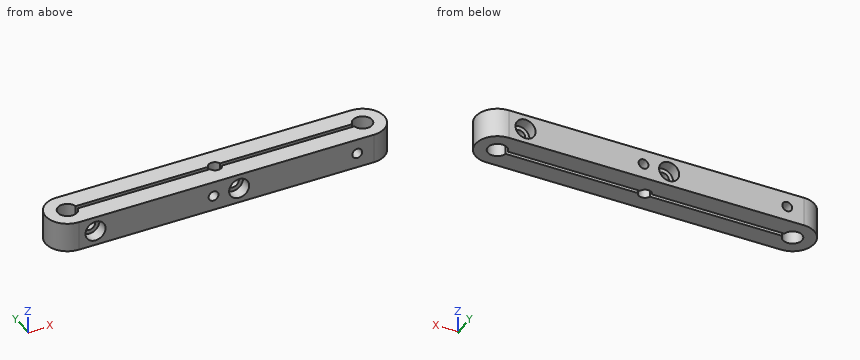
from build123d import *

# Parameters (mm, degrees)
F0_R      = 4.85
F0_R_2    = 3.25
F1_DEPTH  = 15
F3_DEPTH  = 15.001
F4_R      = 2.5
F5_DEPTH  = 22.001
F6_R      = 3
F7_DEPTH  = 10
F8_R      = 3
F9_DEPTH  = 10
F10_R     = 5.1
F11_DEPTH = 6
F12_R     = 5.1
F13_DEPTH = 6


with BuildPart() as f1:
    # F0 (on Top) → F1 (new body)
    with BuildSketch(Plane.XY):
        with BuildLine():
            Line((-75, -11), (0, -11))
            Line((0, -11), (75, -11))
            ThreePointArc((75, -11), (86, 0), (75, 11))
            Line((75, 11), (0, 11))
            Line((0, 11), (-75, 11))
            ThreePointArc((-75, 11), (-86, 0), (-75, -11))
        make_face()
        with Locations((-75, 0)):
            Circle(F0_R, mode=Mode.SUBTRACT)
        Circle(F0_R_2, mode=Mode.SUBTRACT)
        with Locations((75, 0)):
            Circle(F0_R, mode=Mode.SUBTRACT)
    extrude(amount=F1_DEPTH)

    # F2 (on face) → F3 (cut, through all)
    with BuildSketch(Plane.XY.offset(15)):
        Polygon((75, -1), (75, 1), (0, 1), (-75, 1), (-75, -1), (0, -1), align=None)
    extrude(amount=-F3_DEPTH, mode=Mode.SUBTRACT)

    # F4 (on face) → F5 (cut, through all)
    with BuildSketch(Plane.XZ.offset(11)):
        with Locations((-66.5, 7.5)):
            Circle(F4_R)
        with Locations((66.5, 7.5)):
            Circle(F4_R)
        with Locations((-6.5, 7.5)):
            Circle(F4_R)
        with Locations((6.5, 7.5)):
            Circle(F4_R)
    extrude(amount=-F5_DEPTH, mode=Mode.SUBTRACT)

    # F6 (on face) → F7 (cut, through all)
    with BuildSketch(Plane.XZ.offset(11)):
        with Locations((-66.5, 7.5)):
            Circle(F6_R)
        with Locations((6.5, 7.5)):
            Circle(F6_R)
    extrude(amount=-F7_DEPTH, mode=Mode.SUBTRACT)

    # F8 (on face) → F9 (cut, through all)
    with BuildSketch(Plane(origin=(0, 11, 0), x_dir=(-1, 0, 0), z_dir=(0, 1, 0))):
        with Locations((-66.5, 7.5)):
            Circle(F8_R)
        with Locations((6.5, 7.5)):
            Circle(F8_R)
    extrude(amount=-F9_DEPTH, mode=Mode.SUBTRACT)

    # F10 (on face) → F11 (cut)
    with BuildSketch(Plane.XZ.offset(11)):
        with Locations((-66.5, 7.5)):
            Circle(F10_R)
        with Locations((6.5, 7.5)):
            Circle(F10_R)
    extrude(amount=-F11_DEPTH, mode=Mode.SUBTRACT)

    # F12 (on face) → F13 (cut)
    with BuildSketch(Plane(origin=(0, 11, 0), x_dir=(-1, 0, 0), z_dir=(0, 1, 0))):
        with Locations((-66.5, 7.5)):
            Circle(F12_R)
        with Locations((6.5, 7.5)):
            Circle(F12_R)
    extrude(amount=-F13_DEPTH, mode=Mode.SUBTRACT)


solid = f1.part
Geometry check sheet. Reference: the model listing, model coordinates, mm. Give positions to 0.01 mm unless a question says otherwise; leave off trailing zeros. Write each loop counter-clockwise with the first axis right and the second up, starting at its lowest first coordinate (ties: lowest second). Pieces come first, ordered by that corner, then holes.
1) Cross-section at B-B (x = 7). Record the boundary of the cut face in (y, z).
Values follow:
outline: (-11, 0) - (-1, 0) - (-1, 4.54) - (-5, 4.54) - (-5, 2.42) - (-11, 2.42) - close; (-11, 12.58) - (-5, 12.58) - (-5, 10.46) - (-1, 10.46) - (-1, 15) - (-11, 15) - close; (1, 0) - (11, 0) - (11, 5.05) - (1, 5.05) - close; (1, 9.95) - (11, 9.95) - (11, 15) - (1, 15) - close
2) Cross-section at D-D (y = -7.25). Record the boundary of the cut face in (x, z).
Values follow:
outline: (-83.27, 0) - (83.27, 0) - (83.27, 15) - (-83.27, 15) - close; hole circle Ø10.2 at (-66.5, 7.5); hole circle Ø5 at (-6.5, 7.5); hole circle Ø10.2 at (6.5, 7.5); hole circle Ø5 at (66.5, 7.5)
3) Cross-section at A-A (x = -17.5). Record the boundary of the cut face in (y, z).
Values follow:
outline: (-11, 0) - (-1, 0) - (-1, 15) - (-11, 15) - close; (1, 0) - (11, 0) - (11, 15) - (1, 15) - close
4) Thickness scan on line 1 (X direction, y = 6, z = 12); line 2 (X direction, y = 2.25, z = 13.5); line 3 (Y direction, x = 54, z = 13.25). Record the ranges inside material, lowest first.
Values follow:
line 1: x = -84.22 to -8.9, -4.1 to 64.1, 68.9 to 84.22
line 2: x = -85.77 to -79.3, -70.7 to -2.35, 2.35 to 70.7, 79.3 to 85.77
line 3: y = -11 to -1, 1 to 11
5) Cross-section at C-C (z = 7.5). Count the separate pieces of the cut face and the enclosed holes in it, plus the area to 3 significant figures.
Values follow:
separate pieces: 8
enclosed holes: 0
area: 2,690 mm2
